The listing builds one solid part. Answer for the finished solid, in the listing's coordinates (mm). Face numbers are marked on the shaded views. A direction names the side the tool comes from. Round coordinates to 2 decimals unless told otherwise and drop trailing zeros. Write each loop counter-clockwise with the first axis right and the second up, starting at its lowest first coordinate (ties: lowest second). Pieces come first, ordered by that corner, then holes.
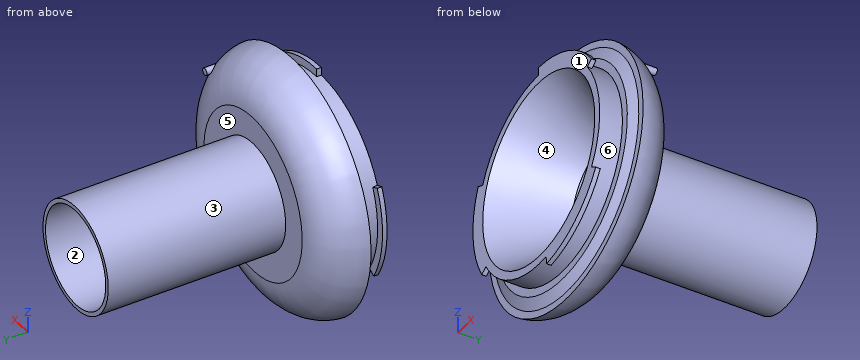
from build123d import *

# Parameters (mm, degrees)
SKETCH1_R           = 21.75
SKETCH1_R_2         = 20
BOSS_EXTRUDE1_DEPTH = 5
SKETCH2_R           = 23.5
SKETCH2_R_2         = 20
BOSS_EXTRUDE2_DEPTH = 1
SKETCH3_R           = 27.5
SKETCH3_R_2         = 20
BOSS_EXTRUDE3_DEPTH = 8
SKETCH4_R           = 11.65
SKETCH4_R_2         = 10.75
BOSS_EXTRUDE4_DEPTH = 40
SKETCH5_R           = 27.5
SKETCH5_R_2         = 11.65
BOSS_EXTRUDE5_DEPTH = 1
BOSS_EXTRUDE6_DEPTH = 1
CIRPATTERN1_COUNT   = 3
FILLET1_R           = 10
SKETCH8_R           = 0.761145908
BOSS_EXTRUDE7_DEPTH = 7
CHAMFER2_SIZE2      = 1
CHAMFER2_SIZE       = 2.475086853


# Some blends are built 0.0001 mm under size
with BuildPart() as part:
    # Sketch1 → Boss-Extrude1 (new body)
    with BuildSketch(Plane(origin=(0, 0, 0), x_dir=(1, 0, 0), z_dir=(0, 1, 0))):
        with Locations(Location((0, 0, 0), (0, 0, 270))):
            Circle(SKETCH1_R)
        with Locations(Location((0, 0, 0), (0, 0, 270))):
            Circle(SKETCH1_R_2, mode=Mode.SUBTRACT)
    boss_extrude1 = extrude(amount=BOSS_EXTRUDE1_DEPTH)

    # Sketch2 → Boss-Extrude2 (add)
    with BuildSketch(Plane(origin=(0, 5, 0), x_dir=(1, 0, 0), z_dir=(0, 1, 0))):
        with Locations(Location((0, 0, 0), (0, 0, 270))):
            Circle(SKETCH2_R)
        with Locations(Location((0, 0, 0), (0, 0, 270))):
            Circle(SKETCH2_R_2, mode=Mode.SUBTRACT)
    extrude(amount=BOSS_EXTRUDE2_DEPTH)

    # Sketch3 → Boss-Extrude3 (add)
    with BuildSketch(Plane(origin=(0, 6, 0), x_dir=(1, 0, 0), z_dir=(0, 1, 0))):
        with Locations(Location((0, 0, 0), (0, 0, 270))):
            Circle(SKETCH3_R)
        with Locations(Location((0, 0, 0), (0, 0, 270))):
            Circle(SKETCH3_R_2, mode=Mode.SUBTRACT)
    extrude(amount=BOSS_EXTRUDE3_DEPTH)



with BuildPart() as body_2:
    # Sketch4 → Boss-Extrude4 (new body)
    with BuildSketch(Plane(origin=(0, 14, 0), x_dir=(1, 0, 0), z_dir=(0, 1, 0))):
        with Locations(Location((0, 0, 0), (0, 0, 270))):
            Circle(SKETCH4_R)
        with Locations(Location((0, 0, 0), (0, 0, 270))):
            Circle(SKETCH4_R_2, mode=Mode.SUBTRACT)
    extrude(amount=BOSS_EXTRUDE4_DEPTH)


with BuildPart() as part_1:
    add(part.part)

    add(body_2.part)  # Boss-Extrude5 merges body 2
    # Sketch5 → Boss-Extrude5 (add)
    with BuildSketch(Plane(origin=(0, 14, 0), x_dir=(1, 0, 0), z_dir=(0, 1, 0))):
        with Locations(Location((0, 0, 0), (0, 0, 270))):
            Circle(SKETCH5_R)
        with Locations(Location((0, 0, 0), (0, 0, 270))):
            Circle(SKETCH5_R_2, mode=Mode.SUBTRACT)
    extrude(amount=BOSS_EXTRUDE5_DEPTH)

    # Sketch6 → Revolve1 (revolve)
    with BuildSketch(Plane.XY, mode=Mode.PRIVATE) as revolve1_sk:
        Polygon((10.75, 14), (20, 0), (20, 14), align=None)
    revolve(revolve1_sk.sketch.rotate(Axis((0, 0, 0), (0, 1, 0)), 90), axis=Axis((0, 0, 0), (0, 1, 0)))

    # Sketch7 → Boss-Extrude6 (add)
    with BuildSketch(Plane.XZ):
        with BuildLine():
            Line((0, 21.75), (0, 23.5))
            ThreePointArc((0, 23.5), (10.5, 21.023796042), (18.787221995, 14.117021277))
            Line((18.787221995, 14.117021277), (17.388173548, 13.065753735))
            ThreePointArc((17.388173548, 13.065753735), (9.718085106, 19.458194209), (0, 21.75))
        make_face()
    boss_extrude6 = extrude(amount=-BOSS_EXTRUDE6_DEPTH)

    # CirPattern1: Boss-Extrude1, Boss-Extrude6 ×3 about axis
    cirpattern1_axis = Axis((0, 0, 0), (0, 1, 0))
    add([boss_extrude1.rotate(cirpattern1_axis, i * 360 / CIRPATTERN1_COUNT) for i in range(1, CIRPATTERN1_COUNT)])
    add([boss_extrude6.rotate(cirpattern1_axis, i * 360 / CIRPATTERN1_COUNT) for i in range(1, CIRPATTERN1_COUNT)])

    # Fillet1
    # the kernel refuses this fillet: 10 mm, written as the material it takes off along each edge
    with BuildSketch(Plane(origin=(0, 15, 0), x_dir=(0, 0, 1), z_dir=(-1, 0, 0))) as fillet1_piece_1:
        with BuildLine():
            CenterArc((17.550125629, -10), FILLET1_R, 5.739170477, 84.260829523)
            Line((17.550125629, 0), (17.550125629, 0.2))
            Line((17.550125629, 0.2), (27.5, 0.2))
            Line((27.5, 0.2), (27.7, 0))
            ThreePointArc((27.7, 0), (27.7, -4.5), (27.698997487, -8.98))
            Line((27.698997487, -8.98), (27.5, -9))
        make_face()
    revolve(axis=Axis((0, 15, 0), (0, 1, 0)), mode=Mode.SUBTRACT)

    # Sketch8 → Boss-Extrude7 (add)
    with BuildSketch(Plane.XZ.offset(-6)):
        with Locations(Location((20.470368468, 14.946483104, 0), (0, 0, 270))):
            Circle(SKETCH8_R)
    extrude(amount=-BOSS_EXTRUDE7_DEPTH)

    # Chamfer2
    chamfer2_edges = [part_1.edges().sort_by_distance(p)[0] for p in [
        (0, 6, -23.5),
    ]]
    chamfer2_side = [part_1.faces().sort_by_distance(p)[0] for p in [
        (0, 6, -23.52),
    ]]
    chamfer(chamfer2_edges, length=CHAMFER2_SIZE - 0.0001, length2=CHAMFER2_SIZE2 - 0.0001, reference=chamfer2_side[0])  # a hair under: the kernel refuses the full size


solid = part_1.part
1. A tool of negligible diameter and unlimited length cuts with its end or side. For the marked faces 4, 5 and 6, from which of +Z, -Z, +X, -X, +Y, -Y can it reach the whole face along a straight path? Write none if from no direction.
Geometry says:
face 4: -Y
face 5: +Y
face 6: none
2. Straight lines are drawn through the part: line 1 along X through (y, z) = (26, 0); line 2 along Z through (x, y) = (0.5, 13); line 3 along Z through (x, y) = (-2.5, 47.5). For each, find the intervals that lie inside material, in ascending order.
Geometry says:
line 1: x = -11.65 to -10.75, 10.75 to 11.65
line 2: z = -23.54 to -11.4, 11.4 to 23.54
line 3: z = -11.38 to -10.46, 10.46 to 11.38
3. For a pull along Z with two mould halves and no side action, classify the marked faces 1, 2 and 3 as released by +Z, released by -Z, zero draft, split by the parting line, or undercut.
Geometry says:
face 1: zero draft
face 2: undercut
face 3: split by the parting line
4. Section B-B on y = 31.5 is taken. Determine the outline of the cut face in (x, z).
Geometry says:
outline: circle Ø23.3 at (0, 0); hole circle Ø21.5 at (0, 0)
5. Given pin 1 (13.5 mm diameter, centred on x = 14.5, z = -17, fed in from +Y); pin 2 (0.8 mm diameter, centred on x = 20.5, z = 14.5, fed in from +Y); pin 3 (3.5 mm diameter, centred on x = -20, z = -5, fed in from +Y); pin 4 (10.5 mm diameter, centred on x = 2, z = -5.5, fed in from +Y), each flat-ended and moving along its own axis, determine where each tip first touches the part or whether it passes through.
Geometry says:
pin 1: stops at y = 15
pin 2: stops at y = 13
pin 3: stops at y = 14.91
pin 4: stops at y = 54
